Autodesk Inventor part; units mm, degrees
ref_plane "YZ Plane" through (0, 0, 0) normal (1, 0, 0) x (0, 1, 0)
ref_plane "XZ Plane" through (0, 0, 0) normal (0, 1, 0) x (-1, 0, 0)
ref_plane "XY Plane" through (0, 0, 0) normal (0, 0, 1) x (1, 0, 0)
sketch "スケッチ1" plane through (0, 0, 0) normal (1, 0, 0) x (0, 1, 0)
  line L0 (-166.8338, 198.3583) -> (193.1662, 198.3583)
  line L1 (193.1662, 198.3583) -> (193.1662, 183.3583)
  line L2 (193.1662, 183.3583) -> (-166.8338, 183.3583)
  line L3 (-166.8338, 183.3583) -> (-166.8338, 198.3583)
  line L4 (-166.8338, 233.3583) -> (-181.8338, 233.3583)
  line L5 (-181.8338, 233.3583) -> (-181.8338, 5.8583)
  line L6 (-181.8338, 5.8583) -> (-166.8338, 5.8583)
  line L7 (-166.8338, 5.8583) -> (-166.8338, 233.3583)
  line L8 (-166.8338, 233.3583) -> (-181.8338, 233.3583)
  line L9 (-181.8338, 233.3583) -> (-181.8338, 218.3583)
  line L10 (-181.8338, 218.3583) -> (-166.8338, 218.3583)
  line L11 (-166.8338, 218.3583) -> (-166.8338, 233.3583)
  line L12 (-116.8338, 183.3583) -> (-101.8338, 183.3583)
  line L13 (-101.8338, 183.3583) -> (-101.8338, 5.8583)
  line L14 (-101.8338, 5.8583) -> (-116.8338, 5.8583)
  line L15 (-116.8338, 5.8583) -> (-116.8338, 183.3583)
  line L16 (193.1662, 183.3583) -> (178.1662, 183.3583)
  line L17 (178.1662, 183.3583) -> (178.1662, 5.8583)
  line L18 (178.1662, 5.8583) -> (193.1662, 5.8583)
  line L19 (193.1662, 5.8583) -> (193.1662, 183.3583)
  circle A0 centre (-141.8338, 138.3583) radius 12.5
  circle A1 centre (-141.8338, 98.3583) radius 18.75
  line L20 (193.1662, 5.8583) -> (-166.8338, 5.8583)
  line L21 (-181.8338, 158.3583) -> (-101.8338, 158.3583)
  line L22 (-101.8338, 78.3583) -> (-181.8338, 78.3583)
  circle A2 centre (-141.8338, 98.3583) radius 20
  line L23 (-124.3338, 198.3583) -> (-124.3338, 183.3583)
  line L24 (-101.8338, 183.3583) -> (-101.8338, 198.3583)
  line L25 (-146.8338, 198.3583) -> (-146.8338, 183.3583)
  line L26 (-166.8338, 205.8583) -> (-181.8338, 205.8583)
  line L27 (-166.8338, 175.8583) -> (-181.8338, 175.8583)
  circle A3 centre (158.1662, 138.3583) radius 12.5
  line L28 (193.1662, 163.3583) -> (178.1662, 163.3583)
  line L29 (170.6662, 198.3583) -> (170.6662, 183.3583)
  line L30 (-166.8338, -186.6417) -> (193.1662, -186.6417)
  line L31 (193.1662, -186.6417) -> (193.1662, -171.6417)
  line L32 (193.1662, -171.6417) -> (-166.8338, -171.6417)
  line L33 (-166.8338, -171.6417) -> (-166.8338, -186.6417)
  line L34 (-166.8338, -221.6417) -> (-181.8338, -221.6417)
  line L35 (-181.8338, -221.6417) -> (-181.8338, 5.8583)
  line L36 (-166.8338, 5.8583) -> (-166.8338, -221.6417)
  line L37 (-166.8338, -221.6417) -> (-181.8338, -221.6417)
  line L38 (-181.8338, -221.6417) -> (-181.8338, -206.6417)
  line L39 (-181.8338, -206.6417) -> (-166.8338, -206.6417)
  line L40 (-166.8338, -206.6417) -> (-166.8338, -221.6417)
  line L41 (-116.8338, -171.6417) -> (-101.8338, -171.6417)
  line L42 (-101.8338, -171.6417) -> (-101.8338, 5.8583)
  line L43 (-116.8338, 5.8583) -> (-116.8338, -171.6417)
  line L44 (193.1662, -171.6417) -> (178.1662, -171.6417)
  line L45 (178.1662, -171.6417) -> (178.1662, 5.8583)
  line L46 (193.1662, 5.8583) -> (193.1662, -171.6417)
  circle A4 centre (-141.8338, -126.6417) radius 12.5
  circle A5 centre (-141.8338, -86.6417) radius 18.75
  line L47 (-181.8338, -146.6417) -> (-101.8338, -146.6417)
  line L48 (-101.8338, -66.6417) -> (-181.8338, -66.6417)
  circle A6 centre (-141.8338, -86.6417) radius 20
  line L49 (-124.3338, -186.6417) -> (-124.3338, -171.6417)
  line L50 (-101.8338, -171.6417) -> (-101.8338, -186.6417)
  line L51 (-146.8338, -186.6417) -> (-146.8338, -171.6417)
  line L52 (-166.8338, -194.1417) -> (-181.8338, -194.1417)
  line L53 (-166.8338, -164.1417) -> (-181.8338, -164.1417)
  circle A7 centre (158.1662, -126.6417) radius 12.5
  line L54 (193.1662, -151.6417) -> (178.1662, -151.6417)
  line L55 (170.6662, -186.6417) -> (170.6662, -171.6417)
  line L56 (193.1662, 158.3583) -> (145.6662, 158.3583)
  line L57 (145.6662, 158.3583) -> (145.6662, 78.3583)
  line L58 (145.6662, 78.3583) -> (193.1662, 78.3583)
  line L59 (193.1662, 78.3583) -> (193.1662, 158.3583)
  line L60 (178.1662, 158.3583) -> (154.1437, 150.1934)
  line L61 (147.3229, 132.1397) -> (178.1662, 78.3583)
  circle A8 centre (-116.8338, 190.8583) radius 1.7
  circle A9 centre (-106.8338, 190.8583) radius 1.7
  circle A10 centre (-109.3338, 178.3583) radius 1.7
  circle A11 centre (-109.3338, 168.3583) radius 1.7
  line L62 (-101.8338, 163.3583) -> (-116.8338, 163.3583)
  line L63 (-99.3338, 198.3583) -> (-99.3338, 183.3583)
  point P0 (0, 0)
  point P1 (-174.3338, 200.8583)
  point P2 (-174.3338, 190.8583)
  point P3 (-174.3338, 180.8583)
  point P4 (-161.8338, 190.8583)
  point P5 (-151.8338, 190.8583)
  point P6 (185.6662, 178.3583)
  point P7 (185.6662, 168.3583)
  point P8 (183.1662, 190.8583)
  point P9 (173.1662, 190.8583)
  point P10 (-109.3338, 183.3583)
  point P11 (193.1662, 190.8583)
  point P12 (-109.3338, 98.3583)
  point P13 (-109.3338, 138.3583)
  point P14 (-174.3338, 138.3583)
  point P15 (-174.3338, 98.3583)
  point P16 (-174.3338, -86.6417)
  point P17 (-109.3338, -86.6417)
  point P18 (-109.3338, -126.6417)
  point P19 (-174.3338, -126.6417)
  point P20 (-174.3338, -169.1417)
  point P21 (-174.3338, -179.1417)
  point P22 (-174.3338, -189.1417)
  point P23 (-161.8338, -179.1417)
  point P24 (-151.8338, -179.1417)
  point P25 (-116.8338, -179.1417)
  point P26 (-106.8338, -179.1417)
  point P27 (-109.3338, -166.6417)
  point P28 (-109.3338, -156.6417)
  point P29 (173.1662, -179.1417)
  point P30 (183.1662, -179.1417)
  point P31 (185.6662, -166.6417)
  point P32 (185.6662, -156.6417)
  point P33 (185.6662, 138.3583)
  point P34 (185.6662, 98.3583)
  point P35 (178.1662, 94.6083)
  point P36 (185.6662, -86.6417)
  point P37 (185.6662, -126.6417)
  point P38 (-116.8338, 158.3583)
  dimension "d0" = 7.5
  dimension "d1" = 7.5
  dimension "d2" = 7.5
  dimension "d3" = 7.5
  dimension "d4" = 10
  dimension "d5" = 10
  dimension "d6" = 5
  dimension "d7" = 10
  dimension "d8" = 7.5
  dimension "d9" = 7.5
  dimension "d10" = 7.5
  dimension "d11" = 10
  dimension "d13" = 7.5
  dimension "d14" = 5
  dimension "d15" = 10
  dimension "d16" = 7.5
  dimension "d17" = 7.5
  dimension "d18" = 10
  dimension "d19" = 10
  dimension "d20" = 7.5
  dimension "d21" = 7.5
  dimension "d22" = 5
  dimension "d23" = 10
  dimension "d24" = 7.5
  dimension "d25" = 7.5
  dimension "d26" = 20
  dimension "d27" = 20
  dimension "d28" = 7.5
  dimension "d29" = 7.5
  dimension "d30" = 20
  dimension "d31" = 7.5
  dimension "d32" = 7.5
  dimension "d33" = 20
  dimension "d34" = 3.4
  dimension "d35" = 3.4
  dimension "d36" = 3.4
  dimension "d37" = 3.4
  dimension "d41" = 5
  dimension "d42" = 15
  dimension "d43" = 5
  dimension "d44" = 22.5
  dimension "d45" = 2.5
extrude "押し出し1" add sketch "スケッチ1" along normal blind 5 contours L0 L24 L2 L23 | L0 L63 L2 L24 | L13 L62 L15 L2
fillet "フィレット1" radius 2 8 edges at (2.5, -124.3338, 198.3583) (2.5, -124.3338, 183.3583) (2.5, -116.8338, 183.3583) (2.5, -116.8338, 163.3583) (2.5, -101.8338, 163.3583) (2.5, -99.3338, 198.3583) (2.5, -99.3338, 183.3583) (2.5, -101.8338, 183.3583)
properties part number "ball_loading_v1_Plate_ASP_F_2" material "ABS プラスチック"
Check sheet for the modelled part. Datum: model origin and axes. Units: mm. A direction names the side the tool comes from. Give positions to 0.01 mm unless a question says otherwise; leave off trailing zeros. Write each loop counter-clockwise with the first axis right and the second up, starting at its lowest first coordinate (ties: lowest second). Pieces come first, ordered by that corner, then holes. Notation, with made-up numbers: (-21, -32) -> (-10, -32) arc R27 ccw to (-10, 5) -> close; hole circle Ø8 at (81.5, 26). An arc over 180 degrees is marked (long way). One line per item, written item: value. Start each with the question number.
Item 1: Draft check along Z on faces 4 (the flat face through (2, -112, 198.358)), 5 (the cylindrical face through (2.465, -108.183, 191.893)), 6 (the cylindrical face through (2.535, -102.435, 163.929)). Enter one of: +Z half, -Z half, draft (parallel to the pull), parting line (faces both ways), or undercut.
Item 2: Section check B-B on y = -108. Record the cut outline in (x, z), then the cut area to 3 significant figures.
Item 3: Section check C-C on z = 192. Record the cut outline in (x, y).
Item 4: Section check D-D on y = -121. Record the cut outline in (x, z), then the cut area to 3 significant figures.
Item 5: Tool access check on faces 1 (the cylindrical face through (2.535, -99.904, 197.757)), 2 (the flat face through (2, -116.834, 173)), 3 (the flat face through (2, -101.834, 174)). Record the directions out of +Z, -Z, +X, -X, +Y, -Y that give a thin tool (end or side, any length) a straight path to the whole face; none if there is none.
Item 6: Gauge pin test, flat ends, axial feed: pin 1 (1.8 mm diameter, centred on x = 3.5, y = -121, fed in from -Z); pin 2 (4 mm diameter, centred on y = -109.33, z = 168.36, fed in from +X); pin 3 (1.5 mm diameter, centred on x = 2, z = 175, fed in from -Y); pin 4 (1.5 mm diameter, centred on x = 3, z = 181.5, fed in from +Y). Record the tip position at first contact, or that the pin passes through.
Item 7: Section check A-A on z = 169. Record the cut outline in (x, y).
Item 8: Material ranges on probe 1 along Z at (x, y) = (2.55, -110.25); probe 2 along Z at (x, y) = (0.45, -109); probe 3 along Y at (x, z) = (2.8, 192), recorded low to high. Write a range as from..to.
Results list:
1. face 4: +Z half
1. face 5: undercut
1. face 6: -Z half
2. outline: (0, 163.36) -> (5, 163.36) -> (5, 167.3) -> (0, 167.3) -> close; (0, 169.41) -> (5, 169.41) -> (5, 177.3) -> (0, 177.3) -> close; (0, 179.41) -> (5, 179.41) -> (5, 189.62) -> (0, 189.62) -> close; (0, 192.1) -> (5, 192.1) -> (5, 198.36) -> (0, 198.36) -> close
2. area: 142 mm²
3. outline: (0, -124.33) -> (5, -124.33) -> (5, -118.09) -> (0, -118.09) -> close; (0, -115.57) -> (5, -115.57) -> (5, -108.09) -> (0, -108.09) -> close; (0, -105.57) -> (5, -105.57) -> (5, -99.33) -> (0, -99.33) -> close
4. outline: (0, 183.36) -> (5, 183.36) -> (5, 198.36) -> (0, 198.36) -> close
4. area: 75.0 mm²
5. face 1: +Z, +X, -X, +Y
5. face 2: -Z, +X, -X, -Y
5. face 3: -Z, +X, -X, +Y
6. pin 1: z = 183.36
6. pin 2: x = 5
6. pin 3: y = -116.83
6. pin 4: y = -101.74
7. outline: (0, -116.83) -> (5, -116.83) -> (5, -110.91) -> (0, -110.91) -> close; (0, -107.76) -> (5, -107.76) -> (5, -101.83) -> (0, -101.83) -> close
8. probe 1: 163.36..166.93, 169.79..176.93, 179.79..198.36
8. probe 2: 163.36..166.69, 170.03..176.69, 180.03..198.36
8. probe 3: -124.33..-118.09, -115.57..-108.09, -105.57..-99.33
